Geometry check sheet. Reference: the model listing, model coordinates, mm. A direction names the side the tool comes from. Coordinates: 2 decimals unless noted, no trailing zeros. Loops run counter-clockwise (first coordinate to the right, second up) from the corner with the lowest first, then second, coordinate; pieces in that order, holes last. Notation, with made-up numbers: (-38.5, -29) - (-3.5, -29) arc R23 ccw to (-3.5, -5) - close; hole circle Ø2 at (44.5, 61). An arc over 180 degrees is marked (long way). One line per item, written item: value.
from build123d import *

# Parameters (mm, degrees)
CHANFREIN1_SIZE         = 0.5
ENL_V_MAT_EXTRU_1_DEPTH = 1.2


with BuildPart() as part:
    # Esquisse1 → Révolution1 (revolve)
    with BuildSketch(Plane.XY):
        Polygon((0, 0), (0, 3), (0.2, 3), (1.7, 1.5), (5, 1.5), (5, 0), align=None)
    revolve(axis=Axis((5, 0, 0), (-1, 0, 0)))

    # Chanfrein1
    chanfrein1_edges = [part.edges().sort_by_distance(p)[0] for p in [
        (5, -1.5, 0),
    ]]
    chamfer(chanfrein1_edges, length=CHANFREIN1_SIZE)

    # Esquisse2 → Enlèv. mat.-Extru.1 (cut)
    with BuildSketch(Plane.ZY):
        Polygon((0, 1.154700538), (-1, 0.577350269), (-1, -0.577350269), (0, -1.154700538), (1, -0.577350269), (1, 0.577350269), align=None)
    extrude(amount=-ENL_V_MAT_EXTRU_1_DEPTH, mode=Mode.SUBTRACT)


solid = part.part
(1) Cross-section at A-A on y = 0. Record the cut outline in (x, z), and give its area (3 significant figures).
Reply:
outline: (0, -3) - (0.2, -3) - (1.7, -1.5) - (4.5, -1.5) - (5, -1) - (5, 1) - (4.5, 1.5) - (1.7, 1.5) - (0.2, 3) - (0, 3) - (0, 1) - (1.2, 1) - (1.2, -1) - (0, -1) - close
area: 15.2 mm2
(2) Cross-section at B-B on x = 4.35. Record the cut outline in (y, z).
Reply:
outline: circle Ø3 at (0, 0)
(3) Access from +Z, -Z, +X, -X, +Y, -Y to the whole of each face (thin tool, end or side, straight path). Record for faces 1 (the face through (5, 0, 0)), 2 (the face through (1, 0, -1)).
Reply:
face 1: +Z, -Z, +X, +Y, -Y
face 2: -X
(4) Release check for a two-part mould opening along Z. For faces 3 (the face through (0.59, 0.86, 0.51)), 4 (the face through (0, 0, 1.3)), 5 (the face through (3.12, -1.5, -0.07)), 6 (the face through (1.2, 0, 0)) record: pulls with the +Z half, pulls with the -Z half, needs draft (parallel to the pull), parting line crosses it, or undercut.
Reply:
face 3: undercut
face 4: needs draft
face 5: parting line crosses it
face 6: undercut
(5) Material ranges on probe 1 along Y at (x, z) = (1.1, 0.6); probe 2 along Z at (x, y) = (0.35, 0.45); probe 3 along Y at (x, z) = (1.5, 0.8), recorded low to high. Write a range as from..to.
Reply:
probe 1: -2.01..-0.81, 0.81..2.01
probe 2: -2.81..-1, 1..2.81
probe 3: -1.5..1.5
(6) Cross-section at C-C on x = 1.55. Record the cut outline in (y, z).
Reply:
outline: circle Ø3.3 at (0, 0)
(7) Go/stop test with flat-tipped pins: pin 1 Ø0.9 at (x, y) = (0.5, -0.5) entering from -Z; pin 2 Ø3 at (x, y) = (2, 0) entering from +Z; pin 3 Ø2 at (x, y) = (2, 2) entering from -Z. Record where each tip stops, or that it passes through.
Reply:
pin 1: z = -3
pin 2: z = 2.7
pin 3: z = -1.43
